Geometry check sheet. Reference: the model listing, model coordinates, mm. A direction names the side the tool comes from. Give positions to 0.01 mm unless a question says otherwise; leave off trailing zeros. Order: outer loops, then holes, each group sorted by start corner. A loop starts at its lowest first (then second) coordinate and runs counter-clockwise, first axis right, second up. Notation, with made-up numbers: M 23.25,-34 L 32.25,-34 A28 ccw 32.25,-2 Z; hole C 12,-36.75 d7. An arc over 180 degrees is marked long. Answer as CSV lines item,"result".
from build123d import *

# Parameters (mm, degrees)
BOSS_EXTRUDE1_DEPTH = 6.35


with BuildPart() as part:
    # Sketch1 → Boss-Extrude1 (new body)
    with BuildSketch(Plane(origin=(0, 0, 0), x_dir=(1, 0, 0), z_dir=(0, 1, 0))):
        with BuildLine():
            Line((2.128963531, 43.884099376), (2.128963531, 57.94662376))
            ThreePointArc((2.128963531, 57.94662376), (11.653963531, 59.797199376), (21.178963531, 57.94662376))
            Line((21.178963531, 57.94662376), (21.178963531, 43.884099376))
            Line((21.178963531, 43.884099376), (35.241487916, 43.884099376))
            ThreePointArc((35.241487916, 43.884099376), (37.092063531, 34.359099376), (35.241487916, 24.834099376))
            Line((35.241487916, 24.834099376), (21.178963531, 24.834099376))
            Line((21.178963531, 24.834099376), (21.178963531, 10.771574991))
            ThreePointArc((21.178963531, 10.771574991), (11.653963531, 8.920999376), (2.128963531, 10.771574991))
            Line((2.128963531, 10.771574991), (2.128963531, 24.834099376))
            Line((2.128963531, 24.834099376), (-11.933560854, 24.834099376))
            ThreePointArc((-11.933560854, 24.834099376), (-13.784136469, 34.359099376), (-11.933560854, 43.884099376))
            Line((-11.933560854, 43.884099376), (2.128963531, 43.884099376))
        make_face()
        with BuildLine():
            Line((11.653963531, 35.806899376), (13.647499485, 35.806899376))
            ThreePointArc((13.647499485, 35.806899376), (14.117763531, 34.359099376), (13.647499485, 32.911299376))
            Line((13.647499485, 32.911299376), (11.653963531, 32.911299376))
            Line((11.653963531, 32.911299376), (9.660427577, 32.911299376))
            ThreePointArc((9.660427577, 32.911299376), (9.190163531, 34.359099376), (9.660427577, 35.806899376))
            Line((9.660427577, 35.806899376), (11.653963531, 35.806899376))
        make_face(mode=Mode.SUBTRACT)
    extrude(amount=BOSS_EXTRUDE1_DEPTH)


solid = part.part
(1) Section check A-A on y = 1. Enter the section's corners in (x, z), then the cut area to 3 significant figures.
The answers:
outline,"M -11.93,-43.88 L 2.13,-43.88 L 2.13,-57.95 A25.44 ccw 21.18,-57.95 L 21.18,-43.88 L 35.24,-43.88 A25.44 ccw 35.24,-24.83 L 21.18,-24.83 L 21.18,-10.77 A25.44 ccw 2.13,-10.77 L 2.13,-24.83 L -11.93,-24.83 A25.44 ccw Z; hole M 9.66,-35.81 L 13.65,-35.81 A2.46 ccw 13.65,-32.91 L 9.66,-32.91 A2.46 ccw Z"
area,"1,520 mm2"
(2) Section check B-B on z = -13.5. Enter the section's corners in (x, y), then the cut area to 3 significant figures.
The answers:
outline,"M 2.13,0 L 21.18,0 L 21.18,6.35 L 2.13,6.35 Z"
area,"121 mm2"
(3) Tool access check on faces 4 (the face through (12, 3, -32.911)), 5 (the face through (28, 3, -24.834)), 6 (the face through (21.179, 3, -51)), 7 (the face through (2.129, 3, -51)). Record the directions out of +Z, -Z, +X, -X, +Y, -Y that give a thin tool (end or side, any length) a straight path to the whole face; none if there is none.
The answers:
face 4,"+Y, -Y"
face 5,"+Z, +X, +Y, -Y"
face 6,"-Z, +X, +Y, -Y"
face 7,"-Z, -X, +Y, -Y"
(4) Material ranges on line 1 (X direction, y = 2.75, z = -19); line 2 (Z direction, x = 24, y = 2.25); line 3 (Z direction, x = 4.5, y = 2.5), recorded low to high.
The answers:
line 1,"x = 2.13 to 21.18"
line 2,"z = -43.88 to -24.83"
line 3,"z = -58.77 to -9.95"
(5) Section check C-C on x = 22.5. Enter the section's corners in (y, z).
The answers:
outline,"M 0,-43.88 L 6.35,-43.88 L 6.35,-24.83 L 0,-24.83 Z"
(6) Draft check along X on faces 1 (the face through (2.129, 3, -18)), 2 (the face through (-5, 3, -24.834)), 3 (the face through (12, 3, -35.807)). Enter one of: +X half, -X half, draft (parallel to the pull), parting line (faces both ways), or undercut.
The answers:
face 1,"-X half"
face 2,"draft"
face 3,"undercut"
(7) Gauge pin test, flat ends, axial feed: P1, Ø1.9, axis at x = 25, y = 3.5, coming from the -Z side; P2, Ø1.5, axis at y = 5, z = -42.5, coming from the +X side; P3, Ø3, axis at y = 4.5, z = -54, coming from the +X side. Record the tip position at first contact, or that the pin passes through.
The answers:
P1,"stops at z = -43.88"
P2,"stops at x = 35.99"
P3,"stops at x = 21.18"
